Input: dimensioned drawing with shaded views. Units: mm. Origin: part minimum x, y, z. A direction names the side the tool comes from. Coordinates: 2 decimals unless noted, no trailing zeros. Write each loop counter-clockwise with the first axis right and the second up, starting at its lowest first coordinate (ties: lowest second). Pieces come first, ordered by that corner, then holes. Notation, with made-up numbers: (11, 81.5) -> (33, 81.5) arc R20 cw to (33, 100.5) -> close; hole circle Ø6 at (-15.75, 31). An arc over 180 degrees is marked (long way). One line per item, written item: value. Start each with the question number.
1. Mould query, pull axis Y, two halves, no side actions, for the marked faces 1, 2 and 3. Classes: released by +Y, released by -Y, zero draft, split by the parting line, or undercut.
2. Section query A-A, the plane x = 2.75. Output: boundary loops of the cut face in (y, z), and give its area (3 significant figures).
3. Section query B-B, the plane y = 2.5. Output: boundary loops of the cut face in (x, z).
4. Section query C-C, the plane z = 4.25. Output: boundary loops of the cut face in (x, y).
5. Line query: line 1 (Z direction, x = 0.6, y = 3.2); line 2 (Z direction, x = 4, y = 2.2); line 3 (X direction, y = 2.25, z = 1.25). Output: solid intervals per line, ascending.
6. Access query for the marked faces 4 and 5. Directions: +Z, -Z, +X, -X, +Y, -Y. A direction counts if a zero-diameter tool reaches every point of the face in a straight line with its end or side. Return the directions, or none.
7. First-contact query: P1, Ø0.8, axis at x = 3, z = 1, coming from the -Y side; P2, Ø2, axis at x = 0.5, y = 4, coming from the +Z side. Flat tips, straight axial feed; report the tip coordinate or a pass-through.
8. Section query D-D, the plane z = 2. Output: boundary loops of the cut face in (x, y).
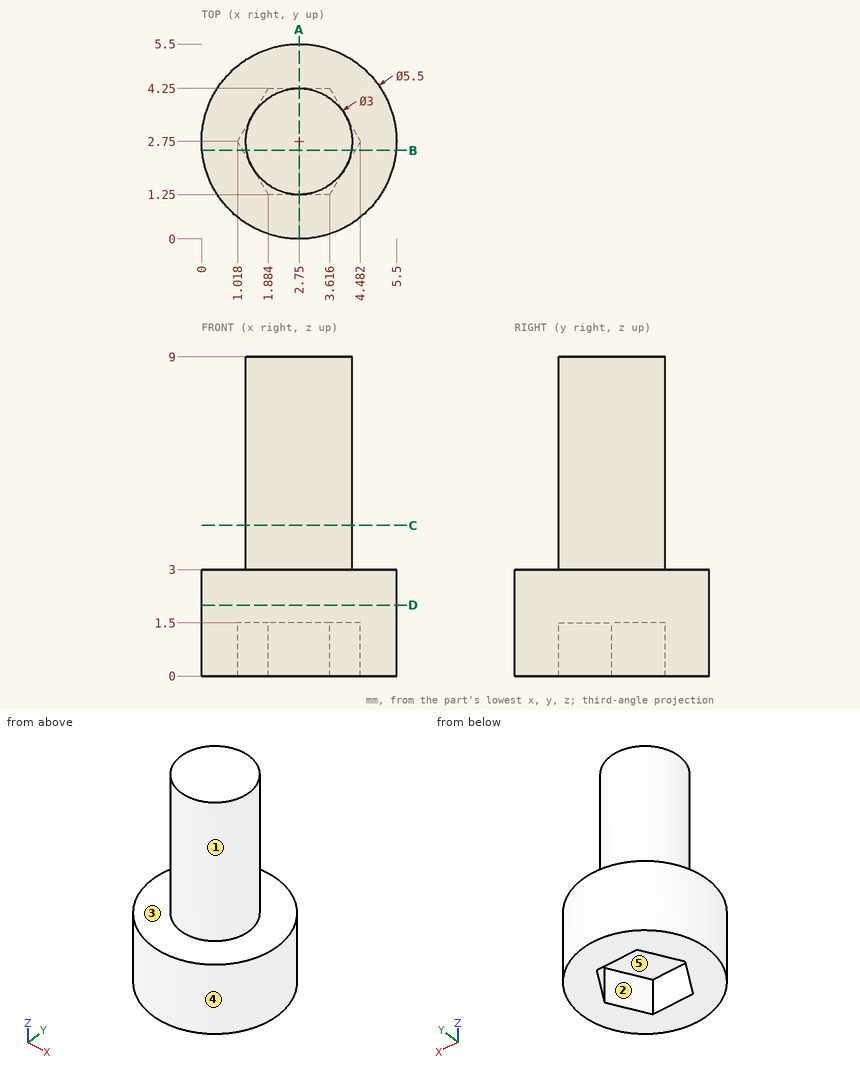
Computed values:
1. face 1: split by the parting line
1. face 2: undercut
1. face 3: zero draft
2. outline: (0, 0) -> (1.25, 0) -> (1.25, 1.5) -> (4.25, 1.5) -> (4.25, 0) -> (5.5, 0) -> (5.5, 3) -> (4.25, 3) -> (4.25, 9) -> (1.25, 9) -> (1.25, 3) -> (0, 3) -> close
2. area: 30.0 mm²
3. outline: (0.01, 0) -> (1.16, 0) -> (1.16, 1.5) -> (4.34, 1.5) -> (4.34, 0) -> (5.49, 0) -> (5.49, 3) -> (4.23, 3) -> (4.23, 9) -> (1.27, 9) -> (1.27, 3) -> (0.01, 3) -> close
4. outline: circle Ø3 at (2.75, 2.75)
5. line 1: z = 0 to 3
5. line 2: z = 1.5 to 9
5. line 3: x = 0.05 to 1.31, 4.19 to 5.45
6. face 4: +Z, -Z
6. face 5: -Z
7. P1: stops at y = 0
7. P2: stops at z = 3
8. outline: circle Ø5.5 at (2.75, 2.75)
